Check sheet for the modelled part. Datum: model origin and axes. Units: mm. A direction names the side the tool comes from. Round coordinates to 2 decimals unless told otherwise and drop trailing zeros. Order: outer loops, then holes, each group sorted by start corner. A loop starts at its lowest first (then second) coordinate and runs counter-clockwise, first axis right, second up. Notation, with made-up numbers: (68, 16.5) -> (127, 16.5) arc R20 cw to (127, 20.5) -> close; hole circle Ø5 at (-4.75, 20.25). An arc over 180 degrees is marked (long way). Answer in a Markdown table with one row per item.
from build123d import *

# Parameters (mm, degrees)
ESBO_O1_W                = 36
ESBO_O1_H                = 22
ESBO_O1_R                = 1.25
RESSALTO_EXTRUS_O1_DEPTH = 2
ESBO_O2_W                = 2
ESBO_O2_H                = 22
RESSALTO_EXTRUS_O2_DEPTH = 6
CORTE_EXTRUS_O1_REACH    = 40.484
ESBO_O3_R                = 1.25


with BuildPart() as part:
    # Esboço1 → Ressalto-extrusão1 (new body)
    with BuildSketch(Plane.XY):
        Rectangle(ESBO_O1_W, ESBO_O1_H)
        with Locations((0, 8)):
            Circle(ESBO_O1_R, mode=Mode.SUBTRACT)
        with Locations((8, 0)):
            Circle(ESBO_O1_R, mode=Mode.SUBTRACT)
        with Locations((0, -8)):
            Circle(ESBO_O1_R, mode=Mode.SUBTRACT)
        with Locations((-8, 0)):
            Circle(ESBO_O1_R, mode=Mode.SUBTRACT)
    extrude(amount=RESSALTO_EXTRUS_O1_DEPTH)

    # Esboço2 → Ressalto-extrusão2 (add)
    with BuildSketch(Plane.XY.offset(2)):
        with Locations((-17, 0)):
            Rectangle(ESBO_O2_W, ESBO_O2_H)
        with Locations((17, 0)):
            Rectangle(ESBO_O2_W, ESBO_O2_H)
    extrude(amount=RESSALTO_EXTRUS_O2_DEPTH)

    # Corte-extrusão1: up to this face of the body (flat: up to its plane)
    corte_extrus_o1_end = Plane(part.part.faces().sort_by_distance((18, 0, 4))[0])
    # Esboço3 → Corte-extrusão1 (cut, up to the picked face)
    with BuildSketch(Plane.ZY.offset(18), mode=Mode.PRIVATE) as corte_extrus_o1_sk1:
        with Locations((4.5, 8)):
            Circle(ESBO_O3_R)
    corte_extrus_o1_tool1 = split(extrude(corte_extrus_o1_sk1.sketch, amount=-CORTE_EXTRUS_O1_REACH, mode=Mode.PRIVATE), bisect_by=corte_extrus_o1_end, keep=Keep.BOTH, mode=Mode.PRIVATE)
    # Esboço3 → Corte-extrusão1 (cut, up to the picked face)
    with BuildSketch(Plane.ZY.offset(18), mode=Mode.PRIVATE) as corte_extrus_o1_sk2:
        with Locations((4.5, -8)):
            Circle(ESBO_O3_R)
    corte_extrus_o1_tool2 = split(extrude(corte_extrus_o1_sk2.sketch, amount=-CORTE_EXTRUS_O1_REACH, mode=Mode.PRIVATE), bisect_by=corte_extrus_o1_end, keep=Keep.BOTH, mode=Mode.PRIVATE)
    add(corte_extrus_o1_tool1.solids().sort_by(Axis((-18, 8, 4.5), (1, 0, 0)))[0], mode=Mode.SUBTRACT)
    add(corte_extrus_o1_tool2.solids().sort_by(Axis((-18, -8, 4.5), (1, 0, 0)))[0], mode=Mode.SUBTRACT)


solid = part.part
Item 1: Set-up check for faces 4 (the flat face through (-1.4, 11, 1.6)), 5 (the flat face through (-16, 0, 5)): record each of +Z, -Z, +X, -X, +Y, -Y from which the full face is reachable in a straight line by a thin tool's end or side.
Result sheet:
| item | result |
|---|---|
| face 4 | +Z, -Z, +X, -X, +Y |
| face 5 | +Z, +Y, -Y |
Item 2: Scan lines: line 1 (Y direction, x = 17.2, z = 4.5); line 2 (X direction, y = 1, z = 4.75); line 3 (Y direction, x = 8, z = 0.4). Record each from-to range of solid material in increasing order. Write a range as [from, to].
Result sheet:
| item | result |
|---|---|
| line 1 | y = [-11, -9.25], [-6.75, 6.75], [9.25, 11] |
| line 2 | x = [-18, -16], [16, 18] |
| line 3 | y = [-11, -1.25], [1.25, 11] |
Item 3: Mould release check, pull along Z, two halves, no side actions. Record for faces 1 (the flat face through (17, 0, 8)), 2 (the cylindrical face through (16.99, -9.22, 4.23)), 3 (the flat face through (16, 0, 5)): pulls with the +Z half, pulls with the -Z half, needs draft (parallel to the pull), parting line crosses it, or undercut.
Result sheet:
| item | result |
|---|---|
| face 1 | pulls with the +Z half |
| face 2 | undercut |
| face 3 | needs draft |
Item 4: Cross-section at A-A (y = -0.75). Record the boundary of the cut face in (x, z).
Result sheet:
| item | result |
|---|---|
| outline | (-18, 0) -> (-9, 0) -> (-9, 2) -> (-16, 2) -> (-16, 8) -> (-18, 8) -> close; (-7, 0) -> (7, 0) -> (7, 2) -> (-7, 2) -> close; (9, 0) -> (18, 0) -> (18, 8) -> (16, 8) -> (16, 2) -> (9, 2) -> close |
Item 5: Depth check by flat-ended pin: P1, Ø10, axis at x = -10, y = 4.5, coming from the +Z side. Enter the tip coordinate at first touch or a pass-through.
Result sheet:
| item | result |
|---|---|
| P1 | stops at z = 2 |
Item 6: Cross-section at D-D (y = 8). Record the boundary of the cut face in (x, z), and give its area (3 significant figures).
Result sheet:
| item | result |
|---|---|
| outline | (-18, 0) -> (-1.25, 0) -> (-1.25, 2) -> (-16, 2) -> (-16, 3.25) -> (-18, 3.25) -> close; (-18, 5.75) -> (-16, 5.75) -> (-16, 8) -> (-18, 8) -> close; (1.25, 0) -> (18, 0) -> (18, 3.25) -> (16, 3.25) -> (16, 2) -> (1.25, 2) -> close; (16, 5.75) -> (18, 5.75) -> (18, 8) -> (16, 8) -> close |
| area | 81.0 mm^2 |
Item 7: Cross-section at B-B (x = 0). Record the boundary of the cut face in (y, z).
Result sheet:
| item | result |
|---|---|
| outline | (-11, 0) -> (-9.25, 0) -> (-9.25, 2) -> (-11, 2) -> close; (-6.75, 0) -> (6.75, 0) -> (6.75, 2) -> (-6.75, 2) -> close; (9.25, 0) -> (11, 0) -> (11, 2) -> (9.25, 2) -> close |
Item 8: Cross-section at C-C (z = 6.5). Record the boundary of the cut face in (x, y), and give its area (3 significant figures).
Result sheet:
| item | result |
|---|---|
| outline | (-18, -11) -> (-16, -11) -> (-16, 11) -> (-18, 11) -> close; (16, -11) -> (18, -11) -> (18, 11) -> (16, 11) -> close |
| area | 88.0 mm^2 |
